from build123d import *

# Parameters (mm, degrees)
SKETCH_R        = 2
PAD_DEPTH       = 10
POCKET004_DEPTH = 1
SKETCH002_W     = 18
SKETCH002_H     = 6
PAD002_DEPTH    = 54
POCKET005_DEPTH = 1
SKETCH003_R     = 14
PAD003_DEPTH    = 18
SKETCH004_R     = 10
POCKET_DEPTH    = 18.001
SKETCH001_W     = 4
SKETCH001_H     = 20
PAD001_DEPTH    = 35.6
SKETCH005_R     = 2
POCKET001_DEPTH = 4
SKETCH006_R     = 2
POCKET002_DEPTH = 4
PAD004_DEPTH    = 6
PAD005_DEPTH    = 6
FILLET_R        = 1


with BuildPart() as part:
    # Sketch → Pad (new body)
    with BuildSketch(Plane.XZ):
        with BuildLine():
            Line((60, 0), (0, 0))
            Line((0, 0), (0, 6))
            Line((12.75, 6), (0, 6))
            Line((12.75, 6), (23.817129, 12.068867))
            ThreePointArc((29, 9), (27.283249, 12.011648), (23.817129, 12.068867))
            Line((29, 9), (29, 4))
            Line((29, 4), (53, 4))
            Line((53, 9), (53, 4))
            ThreePointArc((60, 9), (56.5, 12.5), (53, 9))
            Line((60, 9), (60, 0))
        make_face()
        with Locations((56.5, 9)):
            Circle(SKETCH_R, mode=Mode.SUBTRACT)
        with Locations((25.5, 9)):
            Circle(SKETCH_R, mode=Mode.SUBTRACT)
    extrude(amount=PAD_DEPTH)

    # Sketch007 (on Face14 of Pad) → Pocket004 (cut)
    with BuildSketch(Plane.XZ.offset(10)):
        with BuildLine():
            ThreePointArc((34, 4), (35, 3), (36, 4))
            Line((34, 4), (36, 4))
        make_face()
    extrude(amount=-POCKET004_DEPTH, mode=Mode.SUBTRACT)

    # Sketch002 (on Face13 of Pad) → Pad002 (join)
    with BuildSketch(Plane(origin=(0, 0, 0), x_dir=(1, 0, 0), z_dir=(0, 1, 0))):
        with Locations((9, -3)):
            Rectangle(SKETCH002_W, SKETCH002_H)
    extrude(amount=PAD002_DEPTH)

    # Sketch008 (on Face19 of Pad002) → Pocket005 (cut)
    with BuildSketch(Plane(origin=(0, 0, 0), x_dir=(0, 0, -1), z_dir=(-1, 0, 0))):
        with BuildLine():
            Line((-6, -9), (-6, -11))
            ThreePointArc((-6, -11), (-5, -10), (-6, -9))
        make_face()
    extrude(amount=-POCKET005_DEPTH, mode=Mode.SUBTRACT)

    # Sketch003 (on Face21 of Pad002) → Pad003 (join)
    with BuildSketch(Plane(origin=(0, 0, 0), x_dir=(1, 0, 0), z_dir=(0, 0, -1))):
        with Locations((0, -42)):
            Circle(SKETCH003_R)
    extrude(amount=-PAD003_DEPTH)

    # Sketch004 (on Face21 of Pad002) → Pocket (cut, through all)
    with BuildSketch(Plane(origin=(0, 0, 0), x_dir=(1, 0, 0), z_dir=(0, 0, -1))):
        with Locations((0, -42)):
            Circle(SKETCH004_R)
    extrude(amount=-POCKET_DEPTH, mode=Mode.SUBTRACT)

    # Sketch001 (on Face14 of Pad) → Pad001 (join)
    with BuildSketch(Plane.XZ.offset(7.8)):
        with Locations((2, 16)):
            Rectangle(SKETCH001_W, SKETCH001_H)
    extrude(amount=-PAD001_DEPTH)

    # Sketch005 (on Face26 of Pad001) → Pocket001 (cut)
    with BuildSketch(Plane(origin=(0, 0, 0), x_dir=(0, 0, -1), z_dir=(-1, 0, 0))):
        with Locations((-15, -0.95)):
            Circle(SKETCH005_R)
    extrude(amount=-POCKET001_DEPTH, mode=Mode.SUBTRACT)

    # Sketch006 (on Face26 of Pad001) → Pocket002 (cut)
    with BuildSketch(Plane(origin=(0, 0, 0), x_dir=(0, 0, -1), z_dir=(-1, 0, 0))):
        with Locations((-15, -19.05)):
            Circle(SKETCH006_R)
    extrude(amount=-POCKET002_DEPTH, mode=Mode.SUBTRACT)

    # Sketch009 (on Face25 of Pad001) → Pad004 (join)
    with BuildSketch(Plane.XZ.offset(7.8)):
        with BuildLine():
            Line((4, 16), (4, 6))
            Line((4, 6), (14, 6))
            ThreePointArc((4, 16), (6.928932, 8.928932), (14, 6))
        make_face()
    extrude(amount=-PAD004_DEPTH)

    # Sketch010 (on Face20 of Pad001) → Pad005 (join)
    with BuildSketch(Plane(origin=(0, 27.8, 0), x_dir=(1, 0, 0), z_dir=(0, 1, 0))):
        with BuildLine():
            Line((4, -16), (4, -6))
            Line((4, -6), (13.999971, -6))
            ThreePointArc((13.999971, -6), (6.928922, -8.928942), (4, -16))
        make_face()
    extrude(amount=-PAD005_DEPTH)

    # Fillet
    fillet_edges = [part.edges().sort_by_distance(p)[0] for p in [
        (4, 10, 26),
        (0, 10, 26),
        (2, -7.8, 26),
        (2, 27.8, 26),
        (-14, 42, 18),
        (-10, 42, 18),
    ]]
    fillet(fillet_edges, radius=FILLET_R)


solid = part.part
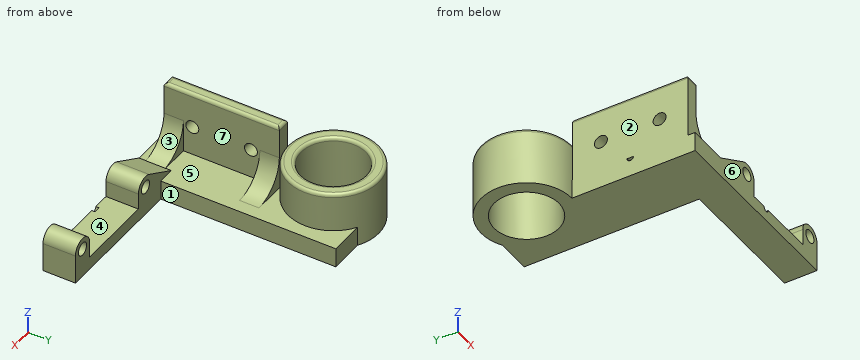
CAD build for the part. Positions are in the model's coordinates, mm. Face numbers are marked on the shaded views. A direction names the side the tool comes from. Give positions to 0.01 mm unless a question says otherwise; leave off trailing zeros. Loops run counter-clockwise (first coordinate to the right, second up) from the corner with the lowest first, then second, coordinate; pieces in that order, holes last. Notation, with made-up numbers: M 45,47.5 L 86,47.5 A19 cw 86,62.5 Z; hole C 12.5,-17.5 d5. An arc over 180 degrees is marked long. Answer in a Markdown table with one row per item. Add a question column.
Item 1: Band-saw the part on C-C on z = 15. Give the cut face in (x, y), then the cut area to 3 significant figures.
Item 2: Band-saw the part on B-B on x = 56.5. Give the cut face in (y, z), then the cut area to 3 significant figures.
Item 3: Probe probe 1 along Z at (x, y) = (2.25, 19.05); probe 2 along X at (y, z) = (42.5, 6.5); probe 3 along X at (y, z) = (42, 5). List the from-to ranges inside material, lowest first.
Item 4: Mould opens along Y. For the marked faces 4, 5, 6 and 7 say: +Y half, -Y half, draft (parallel to the pull), parting line (faces both ways), or undercut.
Item 5: Tool access for the marked faces 1, 2 and 3: list every direction of +Z, -Z, +X, -X, +Y, -Y with a clear straight run to the whole face (end or side of a thin tool).
Item 6: Drop flat-ended pins along their axis: P1, Ø4.5, axis at x = 25.5, z = 9, coming from the +Y side; P2, Ø7.5, axis at y = 0, z = 17.5, coming from the -X side; P3, Ø2, axis at x = 8.5, z = 8.5, coming from the -Y side; P4, Ø12, axis at x = 35.5, y = 11.5, coming from the -Z side. Give the stop position or say it passes through.
Item 7: Band-saw the part on A-A on y = 42. Give the cut face in (x, z).
Item 8: Band-saw the part on D-D on y = 23. Give the cut face in (x, z).
Reply:
| question | item | result |
|---|---|---|
| 1 | outline | C 0,42 d28; M 0,-7.8 L 4.05,-7.8 L 4.05,-1.8 L 4,-1.8 L 4,-1.05 L 0,-1.05 Z; M 0,2.95 L 4,2.95 L 4,17.05 L 0,17.05 Z; M 0,21.05 L 4,21.05 L 4,21.8 L 4.05,21.8 L 4.05,27.8 L 0,27.8 Z; hole C 0,42 d20 |
| 1 | area | 413 mm^2 |
| 2 | outline | M -10,0 L 0,0 L 0,7 L -10,7 Z; M -10,11 L 0,11 L 0,12.5 L -10,12.5 Z |
| 2 | area | 85.0 mm^2 |
| 3 | probe 1 | z = 0 to 13, 17 to 26 |
| 3 | probe 2 | x = -13.99 to -9.99, 9.99 to 13.99 |
| 3 | probe 3 | x = -14 to -10, 10 to 18 |
| 4 | face 4 | draft |
| 4 | face 5 | undercut |
| 4 | face 6 | -Y half |
| 4 | face 7 | undercut |
| 5 | face 1 | +Z, -Z, +X, +Y |
| 5 | face 2 | +Z, -Z, -X, -Y |
| 5 | face 3 | +Z, -Y |
| 6 | P1 | stops at y = 0 |
| 6 | P2 | stops at x = 0 |
| 6 | P3 | stops at y = -7.8 |
| 6 | P4 | passes through |
| 7 | outline | M -14,0 L -10,0 L -10,17 A1 ccw -11,18 L -13,18 A1 ccw -14,17 Z; M 10,0 L 18,0 L 18,6 L 14,6 L 14,17 A1 ccw 13,18 L 11,18 A1 ccw 10,17 Z |
| 8 | outline | M 0,0 L 18,0 L 18,6 L 14,6 A10 cw 4,16 L 4,25 A1 ccw 3,26 L 1,26 A1 ccw 0,25 Z |
